from build123d import *

# Parameters (mm, degrees)
F0_R     = 11
F1_DEPTH = 16.6
F2_R     = 22
F2_R_2   = 11
F3_DEPTH = 2.4
F4_R     = 3.9
F5_DEPTH = 9
F6_R     = 2.75
F7_DEPTH = 25


with BuildPart() as f1:
    # F0 (on Top) → F1 (new body)
    with BuildSketch(Plane.XY):
        Circle(F0_R)
    extrude(amount=F1_DEPTH)

    # F2 (on face) → F3 (join)
    with BuildSketch(Plane.XY.offset(16.6)):
        Circle(F2_R)
        Circle(F2_R_2, mode=Mode.SUBTRACT)
        Circle(F2_R_2)
    extrude(amount=F3_DEPTH)

    # F4 (on face) → F5 (join)
    with BuildSketch(Plane.XY.offset(19)):
        Circle(F4_R)
    extrude(amount=F5_DEPTH)

    # F6 (on face) → F7 (cut)
    with BuildSketch(Plane.XY.offset(19)):
        with Locations((-15.155445, 8.75)):
            Circle(F6_R)
        with Locations((15.155445, 8.75)):
            Circle(F6_R)
        with Locations((0, -17.5)):
            Circle(F6_R)
    extrude(amount=-F7_DEPTH, mode=Mode.SUBTRACT)


solid = f1.part
Read the model definition and answer for the solid it produces. Units are mm, in the model's axes. A direction names the side the tool comes from. Round coordinates to 2 decimals unless told otherwise and drop trailing zeros. Write each loop counter-clockwise with the first axis right and the second up, starting at its lowest first coordinate (ties: lowest second). Pieces come first, ordered by that corner, then holes.
1. The part is cut by section D-D, the plane y = 0. Determine the outline of the cut face in (x, z).
2. The part is cut by section C-C, the plane y = 8.75. Determine the outline of the cut face in (x, z).
3. The part is cut by section A-A, the plane x = 0. Determine the outline of the cut face in (y, z).
4. Straight lines are drawn through the part: L1, parallel to Y at x = 0, z = 17.35; L2, parallel to Z at x = 17, y = -5; L3, parallel to Z at x = -1.5, y = -5. For each, find the intervals that lie inside material, in ascending order.
5. Determine the mould class of faces 3 (the face through (-2.87, 2.64, 23.44)), 4 (the face through (0, 0, 28)), 5 (the face through (17.778, 9.576, 17.817)) for opening direction Y: pulls with the +Y half, pulls with the -Y half, needs draft (parallel to the pull), parting line crosses it, or undercut.
6. Which of the six approach directions +Z, -Z, +X, -X, +Y, -Y give full straight-line access (tool end or side, diameter ignored) to faces 1 (the face through (5, 10, 16.6)), 2 (the face through (-4.769, -21.477, 17.783))?
7. The part is cut by section B-B, the plane y = -17.5. Determine the outline of the cut face in (x, z).
8. Given pin 1 Ø10 at (x, z) = (-16, 18.5) entering from -Y; pin 2 Ø10 at (x, z) = (-13, 11) entering from +Y; pin 3 Ø8 at (y, z) = (-10, 14.5) entering from -X; pin 4 Ø13 at (x, y) = (-3, 9) entering from -Z, each flat-ended and moving along its own axis, determine where each tip first touches the part or whether it passes through.
Values:
1. outline: (-22, 16.6) - (-11, 16.6) - (-11, 0) - (11, 0) - (11, 16.6) - (22, 16.6) - (22, 19) - (3.9, 19) - (3.9, 28) - (-3.9, 28) - (-3.9, 19) - (-22, 19) - close
2. outline: (-20.19, 16.6) - (-17.91, 16.6) - (-17.91, 19) - (-20.19, 19) - close; (-12.41, 16.6) - (-6.67, 16.6) - (-6.67, 0) - (6.67, 0) - (6.67, 16.6) - (12.41, 16.6) - (12.41, 19) - (-12.41, 19) - close; (17.91, 16.6) - (20.19, 16.6) - (20.19, 19) - (17.91, 19) - close
3. outline: (-22, 16.6) - (-20.25, 16.6) - (-20.25, 19) - (-22, 19) - close; (-14.75, 16.6) - (-11, 16.6) - (-11, 0) - (11, 0) - (11, 16.6) - (22, 16.6) - (22, 19) - (3.9, 19) - (3.9, 28) - (-3.9, 28) - (-3.9, 19) - (-14.75, 19) - close
4. L1: y = -22 to -20.25, -14.75 to 22
4. L2: z = 16.6 to 19
4. L3: z = 0 to 19
5. face 3: parting line crosses it
5. face 4: needs draft
5. face 5: undercut
6. face 1: -Z
6. face 2: +Z, -Z
7. outline: (-13.33, 16.6) - (-2.75, 16.6) - (-2.75, 19) - (-13.33, 19) - close; (2.75, 16.6) - (13.33, 16.6) - (13.33, 19) - (2.75, 19) - close
8. pin 1: stops at y = -19.05
8. pin 2: stops at y = 7.55
8. pin 3: stops at x = -20.99
8. pin 4: stops at z = 0
